Can you work these out from the drawing? Everything is in mm from the part's minimum corner. Coordinates: 2 decimals unless noted, no trailing zeros. Order: outer loops, then holes, each group sorted by start corner. A loop starts at its lowest first (then second) coordinate and runs counter-clockwise, first axis right, second up. Notation, with made-up numbers: (4, -22.5) - (23, -22.5) arc R28 ccw to (23, -0.5) - close; hole circle Ø11 at (73, 46). An arc over 180 degrees is marked (long way). Answer as CSV lines item,"result". Start each with the question number.
Q1. I need wall thicknesses on line 1 (X direction, y = 24, z = 20.25); line 2 (Y direction, x = 19, z = 13) (1 decimal); line 3 (Y direction, x = 41, z = 18) (1 decimal). Which ranges of each line are inside material? Lowest first, please.
Q2. Thinking about a two-plate mould opening in Y: for the marked faces 1, 2 and 3, which applies, released by +Y, released by -Y, zero draft, split by the parting line, or undercut?
Q3. Suppose I cut it at A-A (x = 24). Please give me the cut outline in (y, z) (1 decimal).
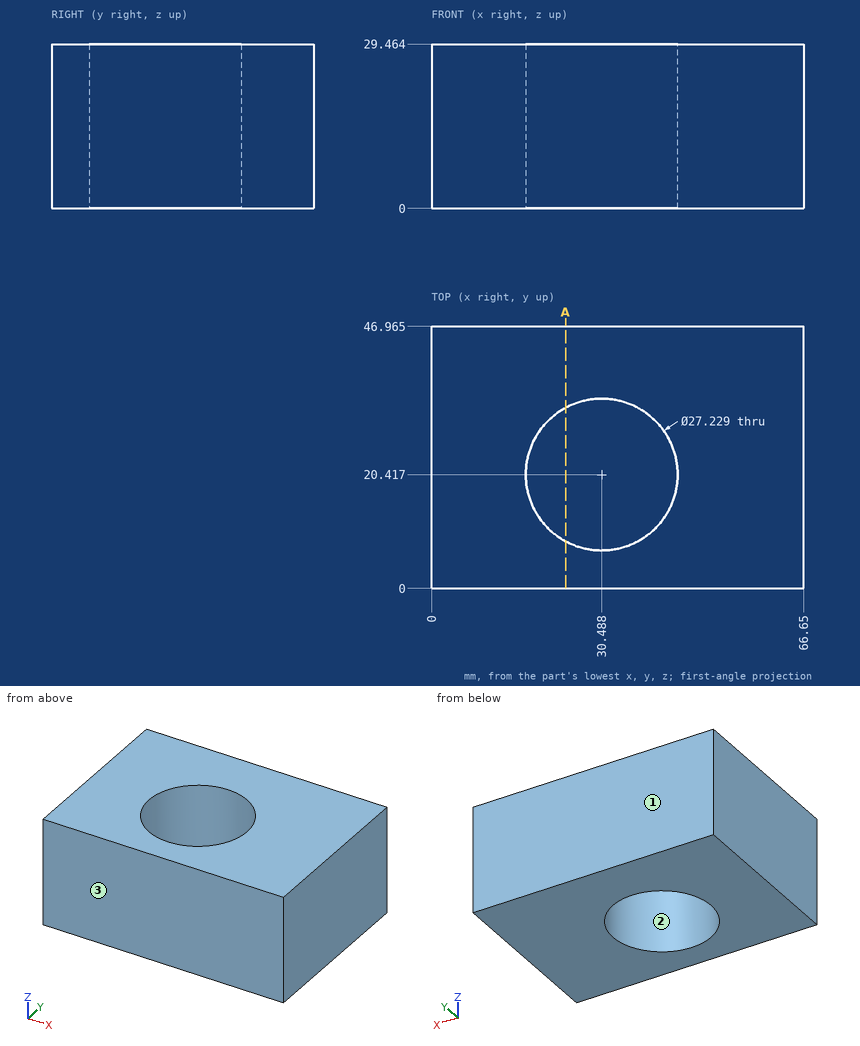
Here are the results:
1,line 1,"x = 0 to 17.35, 43.62 to 66.65"
1,line 2,"y = 0 to 13.1, 27.7 to 47"
1,line 3,"y = 0 to 11.8, 29.1 to 47"
2,face 1,"released by +Y"
2,face 2,"undercut"
2,face 3,"released by -Y"
3,outline,"(0, 0) - (8.4, 0) - (8.4, 29.5) - (0, 29.5) - close; (32.4, 0) - (47, 0) - (47, 29.5) - (32.4, 29.5) - close"
